```python
from build123d import *

# Parameters (mm, degrees)
SKETCH_1_R           = 255
EXTRUDE_1_DEPTH      = 115
CUT_EXTRUDE_1_DEPTH  = 379.516842426
CUT_EXTRUDE_START    = -140
CUT_EXTRUDE_2_DEPTH  = 140
CUT_EXTRUDE_3_DEPTH  = 140
CUT_EXTRUDE_4_DEPTH  = 140
CUT_EXTRUDE_5_DEPTH  = 140
SHELL_1_T            = -1
SKETCH_7_R           = 21.5
CUT_EXTRUDE_6_DEPTH  = 10
CUT_EXTRUDE_7_DEPTH  = 10
CUT_EXTRUDE_8_DEPTH  = 10
SKETCH_10_R          = 6
CUT_EXTRUDE_9_DEPTH  = 10
SKETCH_11_R          = 2.5
CUT_EXTRUDE_10_DEPTH = 10
SKETCH_13_R          = 2.5
CUT_EXTRUDE_11_DEPTH = 10
SKETCH_12_R          = 2.5
CUT_EXTRUDE_12_DEPTH = 10
SKETCH_16_R          = 16
CUT_EXTRUDE_13_DEPTH = 4.5
CUT_EXTRUDE_14_DEPTH = 4.5
SKETCH_18_R          = 3
CUT_EXTRUDE_15_DEPTH = 4.5
SKETCH_19_R          = 3
CUT_EXTRUDE_16_DEPTH = 4.5
SKETCH_20_R          = 3
CUT_EXTRUDE_17_DEPTH = 4.5


with BuildPart() as part:
    # 草图1 → 拉伸1 (new body)
    with BuildSketch(Plane.XY):
        Circle(SKETCH_1_R)
    extrude(amount=EXTRUDE_1_DEPTH)

    # 草图2 → 切除-拉伸1 (cut, through all)
    with BuildSketch(Plane.XY.offset(115)):
        with BuildLine():
            Line((-75, 243.721152139), (-75, 112.168783649))
            Line((-75, 112.168783649), (-149.641016151, -17.113248654))
            Line((-149.641016151, -17.113248654), (-168.970965418, -50.593702892))
            Line((-168.970965418, -50.593702892), (-144.135940052, -93.609228634))
            Line((-144.135940052, -93.609228634), (-216.198889893, -135.214792124))
            ThreePointArc((-216.198889893, -135.214792124), (-238.950435932, 89.037571663), (-75, 243.721152139))
        make_face()
        with BuildLine():
            Line((134.641016151, 8.867513459), (248.568709192, -56.908670786))
            ThreePointArc((248.568709192, -56.908670786), (196.584016918, 162.418361931), (-9, 254.841126979))
            Line((-9, 254.841126979), (-9, 171.63))
            Line((-9, 171.63), (40.670050733, 171.63))
            Line((40.670050733, 171.63), (60, 138.149545762))
            Line((60, 138.149545762), (134.641016151, 8.867513459))
        make_face()
        with BuildLine():
            Line((-173.568709192, -186.812481353), (-59.641016151, -121.036297108))
            Line((-59.641016151, -121.036297108), (89.641016151, -121.036297108))
            Line((89.641016151, -121.036297108), (128.300914685, -121.036297108))
            Line((128.300914685, -121.036297108), (153.135940052, -78.020771366))
            Line((153.135940052, -78.020771366), (225.198889893, -119.626334856))
            ThreePointArc((225.198889893, -119.626334856), (42.366419014, -251.455933595), (-173.568709192, -186.812481353))
        make_face()
    extrude(amount=-CUT_EXTRUDE_1_DEPTH, mode=Mode.SUBTRACT)

    # 草图3 → 切除-拉伸2 (cut)
    with BuildSketch(Plane.XY.offset(115).offset(CUT_EXTRUDE_START)):
        with BuildLine():
            Line((225.198889893, -119.626334856), (215.568709192, -114.066347435))
            Line((215.568709192, -114.066347435), (248.568709192, -56.908670786))
            ThreePointArc((248.568709192, -56.908670786), (238.950435932, -89.037571663), (225.198889893, -119.626334856))
        make_face()
        with BuildLine():
            Line((-9, 254.841126979), (-9, 243.721152139))
            Line((-9, 243.721152139), (-75, 243.721152139))
            ThreePointArc((-75, 243.721152139), (-42.366419014, 251.455933595), (-9, 254.841126979))
        make_face()
        with BuildLine():
            Line((-216.198889893, -135.214792124), (-206.568709192, -129.654804704))
            Line((-206.568709192, -129.654804704), (-173.568709192, -186.812481353))
            ThreePointArc((-173.568709192, -186.812481353), (-196.584016918, -162.418361931), (-216.198889893, -135.214792124))
        make_face()
    extrude(amount=CUT_EXTRUDE_2_DEPTH, mode=Mode.SUBTRACT)

    # 草图4 → 切除-拉伸3 (cut)
    with BuildSketch(Plane(origin=(37.5, -64.951905284, 0), x_dir=(0.8660254037844386, 0.5000000000000002, 0), z_dir=(0.5000000000000002, -0.8660254037844386, 0))):
        Polygon((-171.521152139, 115), (-243.721152139, 115), (-243.721152139, 52.281731212), align=None)
    extrude(amount=-CUT_EXTRUDE_3_DEPTH, mode=Mode.SUBTRACT)

    # 草图5 → 切除-拉伸4 (cut)
    with BuildSketch(Plane(origin=(37.5, 64.951905284, 0), x_dir=(-0.8660254037844387, 0.4999999999999999, 0), z_dir=(0.4999999999999999, 0.8660254037844387, 0))):
        Polygon((-171.521152139, 115), (-243.721152139, 115), (-243.721152139, 52.281731212), align=None)
    extrude(amount=-CUT_EXTRUDE_4_DEPTH, mode=Mode.SUBTRACT)

    # 草图6 → 切除-拉伸5 (cut)
    with BuildSketch(Plane.ZY.offset(75)):
        Polygon((115, 171.521152139), (115, 243.721152139), (52.281731212, 243.721152139), align=None)
    extrude(amount=-CUT_EXTRUDE_5_DEPTH, mode=Mode.SUBTRACT)

    # 抽壳1
    shell_1_openings = [part.faces().sort_by_distance(p)[0] for p in [
        (0, 0, 0),
    ]]
    offset(amount=SHELL_1_T, openings=shell_1_openings, kind=Kind.INTERSECTION)

    # 草图7 → 切除-拉伸6 (cut)
    with BuildSketch(Plane(origin=(-9, 0, 0), x_dir=(0, 0, -1), z_dir=(1, 0, 0))):
        with Locations(Location((-35.3, 208.831152139, 0), (0, 0, 90))):
            Circle(SKETCH_7_R)
    extrude(amount=-CUT_EXTRUDE_6_DEPTH, mode=Mode.SUBTRACT)

    # 草图8 → 切除-拉伸7 (cut)
    with BuildSketch(Plane(origin=(4.5, 7.794228634, 0), x_dir=(0.8660254037844387, -0.5, 0), z_dir=(-0.5, -0.8660254037844387, 0))):
        with BuildLine():
            Line((202.443951117, 55.829336646), (184.789521579, 73.483766184))
            Line((184.789521579, 73.483766184), (174.182919861, 62.877164466))
            Line((174.182919861, 62.877164466), (190.509645151, 46.550439177))
            ThreePointArc((190.509645151, 46.550439177), (222.027914903, 18.326625187), (202.443951117, 55.829336646))
        make_face()
    extrude(amount=-CUT_EXTRUDE_7_DEPTH, mode=Mode.SUBTRACT)

    # 草图9 → 切除-拉伸8 (cut)
    with BuildSketch(Plane(origin=(4.5, -7.794228634, 0), x_dir=(-0.8660254037844388, -0.4999999999999996, 0), z_dir=(-0.4999999999999996, 0.8660254037844388, 0))):
        with BuildLine():
            Line((202.443951117, 55.829336646), (184.789521579, 73.483766184))
            Line((184.789521579, 73.483766184), (174.182919861, 62.877164466))
            Line((174.182919861, 62.877164466), (190.509645151, 46.550439177))
            ThreePointArc((190.509645151, 46.550439177), (222.027914903, 18.326625187), (202.443951117, 55.829336646))
        make_face()
    extrude(amount=-CUT_EXTRUDE_8_DEPTH, mode=Mode.SUBTRACT)

    # 草图10 → 切除-拉伸9 (cut)
    with BuildSketch(Plane.XY.offset(115)):
        with Locations((-22.5, 60.111069989)):
            Circle(SKETCH_10_R)
        with Locations((-40.807713659, -49.54110658)):
            Circle(SKETCH_10_R)
        with Locations((63.307713659, -10.56996341)):
            Circle(SKETCH_10_R)
    extrude(amount=-CUT_EXTRUDE_9_DEPTH, mode=Mode.SUBTRACT)

    # 草图11 → 切除-拉伸10 (cut)
    with BuildSketch(Plane(origin=(-9, 0, 0), x_dir=(0, 0, -1), z_dir=(1, 0, 0))):
        with Locations(Location((-7.30433866, 208.832756681, 0), (0, 0, 90))):
            Circle(SKETCH_11_R)
    extrude(amount=-CUT_EXTRUDE_10_DEPTH, mode=Mode.SUBTRACT)

    # 草图13 → 切除-拉伸11 (cut)
    with BuildSketch(Plane(origin=(4.5, -7.794228634, 0), x_dir=(-0.8660254037844389, -0.4999999999999995, 0), z_dir=(-0.4999999999999995, 0.8660254037844389, 0))):
        with Locations((208.832756681, 7.30433866)):
            Circle(SKETCH_13_R)
    extrude(amount=-CUT_EXTRUDE_11_DEPTH, mode=Mode.SUBTRACT)

    # 草图12 → 切除-拉伸12 (cut)
    with BuildSketch(Plane(origin=(4.5, 7.794228634, 0), x_dir=(0.8660254037844386, -0.4999999999999999, 0), z_dir=(-0.49999999999999994, -0.8660254037844387, 0))):
        with Locations((208.832756681, 7.30433866)):
            Circle(SKETCH_12_R)
    extrude(amount=-CUT_EXTRUDE_12_DEPTH, mode=Mode.SUBTRACT)

    # 草图16 → 切除-拉伸13 (cut)
    with BuildSketch(Plane(origin=(104.820508076, 60.518148554, 0), x_dir=(0, 0, -1), z_dir=(0.8660254037844385, 0.5000000000000004, 0))):
        with Locations(Location((-75, -1.699085315, 0), (0, 0, 90))):
            Circle(SKETCH_16_R)
    extrude(amount=-CUT_EXTRUDE_13_DEPTH, mode=Mode.SUBTRACT)

    # 草图17 → 切除-拉伸14 (cut)
    with BuildSketch(Plane(origin=(-9, 0, 0), x_dir=(0, 0, -1), z_dir=(1, 0, 0))):
        with BuildLine():
            Line((-55.907885828, 202.70211945), (-73.782506819, 185.270662567))
            Line((-73.782506819, 185.270662567), (-63.309864805, 174.531772063))
            Line((-63.309864805, 174.531772063), (-46.779507597, 190.652293392))
            ThreePointArc((-46.779507597, 190.652293392), (-18.162328595, 221.813841337), (-55.907885828, 202.70211945))
        make_face()
    extrude(amount=-CUT_EXTRUDE_14_DEPTH, mode=Mode.SUBTRACT)

    # 草图18 → 切除-拉伸15 (cut)
    with BuildSketch(Plane(origin=(0, 171.63, 0), x_dir=(-1, 0, 0), z_dir=(0, 1, 0))):
        with Locations(Location((4, 74.905446684, 0), (0, 0, 90))):
            Circle(SKETCH_18_R)
    extrude(amount=-CUT_EXTRUDE_15_DEPTH, mode=Mode.SUBTRACT)

    # 草图19 → 切除-拉伸16 (cut)
    with BuildSketch(Plane(origin=(148.635940052, -85.815, 0), x_dir=(0, 0, -1), z_dir=(0.8660254037844388, -0.49999999999999983, 0))):
        with Locations(Location((-74.905446684, 4, 0), (0, 0, 90))):
            Circle(SKETCH_19_R)
    extrude(amount=-CUT_EXTRUDE_16_DEPTH, mode=Mode.SUBTRACT)

    # 草图20 → 切除-拉伸17 (cut)
    with BuildSketch(Plane(origin=(-148.635940052, -85.815, 0), x_dir=(0, 0, 1), z_dir=(-0.866025403784438, -0.5000000000000009, 0))):
        with Locations(Location((74.905446684, -4, 0), (0, 0, 270))):
            Circle(SKETCH_20_R)
    extrude(amount=-CUT_EXTRUDE_17_DEPTH, mode=Mode.SUBTRACT)


solid = part.part
```
Verification items for the finished model (mm, model axes). A direction names the side the tool comes from. Round coordinates to 2 decimals unless told otherwise and drop trailing zeros. Order: outer loops, then holes, each group sorted by start corner. A loop starts at its lowest first (then second) coordinate and runs counter-clockwise, first axis right, second up. Notation, with made-up numbers: (58, 1) - (75, 1) arc R7 ccw to (75, 5) - close; hole circle Ø5 at (57, -12.5). An arc over 180 degrees is marked (long way). Use CSV: the item, a comma, the result in double quotes. Start each with the question number.
1) Mould release check, pull along Z, two halves, no side actions. Record for faces 1 (the flat face through (-173.549, -111.746, 57.798)), 2 (the flat face through (-163.04, -105.09, 64.53)), 3 (the flat face through (-158.42, -140.479, 82.478)), 4 (the flat face through (-9.493, 179.976, 68.619)): +Z half, -Z half, draft (parallel to the pull), parting line (faces both ways), or undercut.
2) Go/stop test with flat-tipped pins: P1, Ø21.5, axis at y = 194.5, z = 83, coming from the +X side; P2, Ø2, axis at x = 95.5, y = 6.5, coming from the -Z side; P3, Ø2, axis at x = 132, z = 94.5, coming from the +Y side. Record where each tip stops, or that it passes through.
3) Thickness scan on L1, parallel to Y at x = 25.5, z = 13.5; L2, parallel to X at y = -83, z = 58; L3, parallel to X at y = 174, z = 14.5. Record the ranges inside material, lowest first.
4) Access from +Z, -Z, +X, -X, +Y, -Y to the whole of each face (thin tool, end or side, straight path). Record for faces 5 (the flat face through (-42, 242.721, 26)), 6 (the cylindrical face through (-186.954, -118.9, 17.826)), 7 (the cylindrical face through (-9.49, 221.14, 17.67)), 8 (the flat face through (15, 171.63, 58)), 9 (the flat face through (33, -121.036, 58)).
5) Section check C-C, the plane x = 79. Record the cut outline in (y, z).
6) Section check A-A, the plane x = -22.5. Record the cut outline in (y, z).
7) Section check D-D, the plane y = 146. Record the cut outline in (x, z).
Answers:
1,face 1,"draft"
1,face 2,"undercut"
1,face 3,"-Z half"
1,face 4,"undercut"
2,P1,"stops at x = -9"
2,P2,"stops at z = 114"
2,P3,"stops at y = 15.17"
3,L1,"y = -121.04 to -120.04, 170.63 to 171.63"
3,L2,"x = -150.26 to -149.11, 149.11 to 150.26, 224.14 to 225.9"
3,L3,"x = -75 to -74, -10 to -9"
4,face 5,"-Z"
4,face 6,"none"
4,face 7,"+X"
4,face 8,"+Z, -Z, +X, +Y"
4,face 9,"+Z, -Z, +X, -Y"
5,outline,"(-121.04, 0) - (-120.04, 0) - (-120.04, 114) - (103.24, 114) - (103.24, 0) - (105.24, 0) - (105.24, 115) - (-121.04, 115) - close"
6,outline,"(-121.04, 0) - (-120.04, 0) - (-120.04, 114) - (54.11, 114) - (54.11, 115) - (-121.04, 115) - close; (66.11, 114) - (171.15, 114) - (242.72, 51.83) - (242.72, 0) - (243.72, 0) - (243.72, 52.28) - (171.52, 115) - (66.11, 115) - close"
7,outline,"(-75, 0) - (-74, 0) - (-74, 114) - (54.31, 114) - (54.31, 0) - (55.47, 0) - (55.47, 115) - (-75, 115) - close"
